The model under review builds one solid part; all positions refer to its coordinate system, in mm. Face numbers are marked on the shaded views. A direction names the side the tool comes from. Coordinates: 2 decimals unless noted, no trailing zeros. Loops run counter-clockwise (first coordinate to the right, second up) from the corner with the lowest first, then second, coordinate; pieces in that order, holes last. Notation, with made-up numbers: M 83,75 L 140,75 A28 cw 140,93 Z; hole C 81.25,14 d8. An arc over 180 degrees is marked long. Return JSON: item names as keys, results as strings.
```python
from build123d import *

# Parameters (mm, degrees)
BOSS_EXTRUDE1_START     = -3
SKETCH1_R               = 42
BOSS_EXTRUDE1_DEPTH     = 24
BOSS_EXTRUDE2_START     = -3
BOSS_EXTRUDE2_DEPTH     = 24
CUT_EXTRUDE1_START      = -3
CUT_EXTRUDE1_DEPTH      = 22.8
CUT_EXTRUDE2_DEPTH      = 169.170182404
CUT_EXTRUDE2_DEPTH_BACK = 169.170182404
SKETCH4_R               = 40.8
BOSS_EXTRUDE3_START     = 21
SKETCH5_R               = 16
BOSS_EXTRUDE3_DEPTH     = 6.2
CUT_EXTRUDE3_START      = 19.8
SKETCH6_R               = 14.8
CUT_EXTRUDE3_DEPTH      = 6.2
BOSS_EXTRUDE4_START     = 9
SKETCH7_R               = 3.5
BOSS_EXTRUDE4_DEPTH     = 10.8
CUT_EXTRUDE4_DEPTH      = 170.05635229
CUT_EXTRUDE4_DEPTH_BACK = 170.05635229
SKETCH8_R               = 1.725


with BuildPart() as part:
    # Sketch1 → Boss-Extrude1 (new body)
    with BuildSketch(Plane.XY.offset(BOSS_EXTRUDE1_START)):
        Circle(SKETCH1_R)
    extrude(amount=BOSS_EXTRUDE1_DEPTH)

    # Sketch2 → Boss-Extrude2 (add)
    with BuildSketch(Plane.XY.offset(BOSS_EXTRUDE2_START)):
        Polygon((-38.5, 0), (-38.3954, -1.3297), (-38.084, -2.6266), (-37.5736, -3.8589), (-36.8766, -4.9962), (-36.0104, -6.0104), (-34.9962, -6.8766), (-33.8589, -7.5736), (-32.6266, -8.084), (-31.3297, -8.3954), (27.497, -15.803), (126.2456, -23.7045), (130, -24), (133.7544, -23.7045), (137.4164, -22.8254), (140.8958, -21.3842), (144.1068, -19.4164), (146.9706, -16.9706), (149.4164, -14.1068), (151.3842, -10.8958), (152.8254, -7.4164), (161.0653, 16.657), (161.3767, 17.9539), (161.4813, 19.2836), (161.3767, 20.6133), (161.0653, 21.9103), (160.5549, 23.1425), (159.858, 24.2798), (158.9917, 25.294), (155.294, 28.9917), (154.2798, 29.858), (149.9962, 32.8574), (148.8589, 33.5543), (144.1195, 35.7643), (142.8872, 36.2748), (137.8361, 37.6282), (136.5391, 37.9396), (131.3297, 38.3954), (130, 38.5), (0, 38.5), (-1.3297, 38.3954), (-6.5391, 37.9396), (-7.8361, 37.6282), (-12.8872, 36.2748), (-14.1195, 35.7643), (-18.8589, 33.5543), (-19.9962, 32.8574), (-24.2798, 29.858), (-25.294, 28.9917), (-28.9917, 25.294), (-29.858, 24.2798), (-32.8574, 19.9962), (-33.5543, 18.8589), (-35.7643, 14.1195), (-36.2748, 12.8872), (-37.6282, 7.8361), (-37.9396, 6.5391), (-38.3954, 1.3297), align=None)
    extrude(amount=BOSS_EXTRUDE2_DEPTH)

    # Sketch3 → Cut-Extrude1 (cut)
    with BuildSketch(Plane.XY.offset(CUT_EXTRUDE1_START)):
        Polygon((-37.3, 0), (-37.2101, -1.142), (-36.9427, -2.2558), (-36.5043, -3.3141), (-35.9058, -4.2908), (-35.1619, -5.1619), (-34.2908, -5.9058), (-33.3141, -6.5043), (-32.2558, -6.9427), (-31.142, -7.2101), (27.6848, -14.6178), (126.4333, -22.5193), (130, -22.8), (133.5667, -22.5193), (137.0456, -21.6841), (140.351, -20.3149), (143.4015, -18.4456), (146.122, -16.122), (148.4456, -13.4015), (150.3149, -10.351), (151.6841, -7.0456), (159.924, 17.0278), (160.1915, 18.1417), (160.2813, 19.2836), (160.1915, 20.4256), (159.924, 21.5395), (159.4857, 22.5978), (158.8872, 23.5745), (158.1432, 24.4455), (154.4455, 28.1432), (153.5745, 28.8872), (149.2908, 31.8866), (148.3141, 32.4851), (143.5747, 34.6951), (142.5164, 35.1335), (137.4653, 36.4869), (136.3514, 36.7544), (131.142, 37.2101), (130, 37.3), (0, 37.3), (-1.142, 37.2101), (-6.3514, 36.7544), (-7.4653, 36.4869), (-12.5164, 35.1335), (-13.5747, 34.6951), (-18.3141, 32.4851), (-19.2908, 31.8866), (-23.5745, 28.8872), (-24.4455, 28.1432), (-28.1432, 24.4455), (-28.8872, 23.5745), (-31.8866, 19.2908), (-32.4851, 18.3141), (-34.6951, 13.5747), (-35.1335, 12.5164), (-36.4869, 7.4653), (-36.7544, 6.3514), (-37.2101, 1.142), align=None)
    extrude(amount=CUT_EXTRUDE1_DEPTH, mode=Mode.SUBTRACT)

    # Sketch4 → Cut-Extrude2 (cut, two sides: drawn at the far end of the back side and taken through both)
    with BuildSketch(Plane.XY.offset(-CUT_EXTRUDE2_DEPTH_BACK)):
        Circle(SKETCH4_R)
    extrude(amount=CUT_EXTRUDE2_DEPTH + CUT_EXTRUDE2_DEPTH_BACK, mode=Mode.SUBTRACT)

    # Sketch5 → Boss-Extrude3 (add)
    with BuildSketch(Plane.XY.offset(BOSS_EXTRUDE3_START)):
        with Locations((130, 0)):
            Circle(SKETCH5_R)
    extrude(amount=BOSS_EXTRUDE3_DEPTH)

    # Sketch6 → Cut-Extrude3 (cut)
    with BuildSketch(Plane.XY.offset(CUT_EXTRUDE3_START)):
        with Locations((130, 0)):
            Circle(SKETCH6_R)
    extrude(amount=CUT_EXTRUDE3_DEPTH, mode=Mode.SUBTRACT)

    # Sketch7 → Boss-Extrude4 (add)
    with BuildSketch(Plane.XY.offset(BOSS_EXTRUDE4_START)):
        with Locations(Location((50, 0, 0), (0, 0, 180))):
            Circle(SKETCH7_R)
        with Locations(Location((90, 0, 0), (0, 0, 180))):
            Circle(SKETCH7_R)
    extrude(amount=BOSS_EXTRUDE4_DEPTH)

    # Sketch8 → Cut-Extrude4 (cut, two sides: drawn at the far end of the back side and taken through both)
    with BuildSketch(Plane.XY.offset(-CUT_EXTRUDE4_DEPTH_BACK)):
        with Locations((50, 0)):
            Circle(SKETCH8_R)
        with Locations((90, 0)):
            Circle(SKETCH8_R)
    extrude(amount=CUT_EXTRUDE4_DEPTH + CUT_EXTRUDE4_DEPTH_BACK, mode=Mode.SUBTRACT)


solid = part.part
```
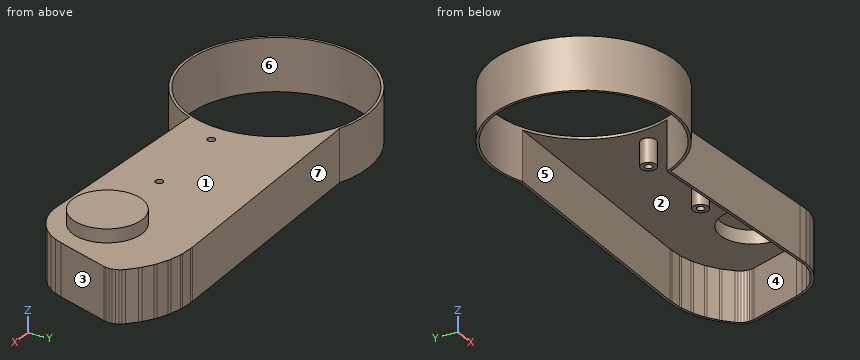
1. Add section A-A on x = 0. Give the boundary of the cut face in (y, z), plus the area to 3 significant figures.
Check values:
{"outline": "M -42,-3 L -40.8,-3 L -40.8,21 L -42,21 Z; M 40.8,-3 L 42,-3 L 42,21 L 40.8,21 Z", "area": "57.6 mm²"}
2. Insertion check: pin 1 Ø6 at (y, z) = (7, 7.5) entering from +X; pin 2 Ø23.5 at (x, y) = (131, 0) entering from -Z; pin 3 Ø5.5 at (x, y) = (89.5, 1.5) entering from -Z. Each pin has a flat end and moves straight along its axis. Give the tip position at first contact, or say it passes through.
Check values:
{"pin 1": "x = 158.79", "pin 2": "z = 26", "pin 3": "z = 9"}
3. To check wall thickness, follow line 1 (Y direction, x = 90, z = 15.75) (3 decimals); line 2 (X direction, y = 1.5, z = 13); line 3 (Y direction, x = 50, z = 16) (3 decimals). State the ranges of each line that lie inside material, in increasing order.
Check values:
{"line 1": "-20.804 to -19.604, -3.5 to -1.725, 1.725 to 3.5, 37.3 to 38.5", "line 2": "-41.97 to -40.77, 46.84 to 49.15, 50.85 to 53.16, 86.84 to 89.15, 90.85 to 93.16, 154.61 to 155.88", "line 3": "-17.604 to -16.403, -3.5 to -1.725, 1.725 to 3.5, 37.3 to 38.5"}
4. Add section D-D on y = -26. Give the boundary of the cut face in (x, z), plus the area to 3 significant figures.
Check values:
{"outline": "M -32.98,-3 L -31.44,-3 L -31.44,21 L -32.98,21 Z; M 31.44,-3 L 32.98,-3 L 32.98,21 L 31.44,21 Z", "area": "74.0 mm²"}
5. Add section C-C on y = 9.5. Give the boundary of the cut face in (x, z), plus the area to 3 significant figures.
Check values:
{"outline": "M -40.91,-3 L -39.68,-3 L -39.68,21 L -40.91,21 Z; M 39.68,19.8 L 118.65,19.8 L 118.65,26 L 141.35,26 L 141.35,19.8 L 157.35,19.8 L 157.35,-3 L 158.62,-3 L 158.62,21 L 142.87,21 L 142.87,27.2 L 117.13,27.2 L 117.13,21 L 39.68,21 Z", "area": "220 mm²"}
6. Add section B-B on z = 13. State how many separate pieces and enclosed holes the cut face has, plus the area to 3 significant figures.
Check values:
{"separate pieces": "3", "enclosed holes": "3", "area": "654 mm²"}
7. The part is to be moulded in two halves that separate along X. For the marked faces 1, 2, 3 and 4, say which applies: released by +X, released by -X, zero draft, split by the parting line, or undercut.
Check values:
{"face 1": "zero draft", "face 2": "undercut", "face 3": "released by +X", "face 4": "undercut"}
8. Machinability: for the marked faces 5, 6 and 7, which of the approach directions +Z, -Z, +X, -X, +Y, -Y give a long, thin tool a straight path to every point of the face, cutting with its end or side? Answer none if there is none.
Check values:
{"face 5": "-Z", "face 6": "+Z, -Z", "face 7": "+Z, -Z, +X, +Y"}
